Autodesk Inventor part; units mm, degrees
ref_plane "YZ Plane" through (0, 0, 0) normal (1, 0, 0) x (0, 1, 0)
ref_plane "XZ Plane" through (0, 0, 0) normal (0, 1, 0) x (-1, 0, 0)
ref_plane "XY Plane" through (0, 0, 0) normal (0, 0, 1) x (1, 0, 0)
sketch "Sketch1" plane through (0, 0, 0) normal (0, 0, 1) x (1, 0, 0)
  line L0 (-250, 0) -> (250, 0) construction
  line L1 (-250, -50) -> (250, -50)
  line L2 (250, 50) -> (-250, 50)
  arc A0 (-250, 50) -> (-250, -50) centre (-250, 0) ccw
  arc A1 (250, -50) -> (250, 50) centre (250, 0) ccw
  circle A2 centre (-250, 0) radius 25
  circle A3 centre (0, 0) radius 25
  circle A4 centre (250, 0) radius 25
  circle A5 centre (-125, 0) radius 25
  circle A6 centre (125, 0) radius 25
  dimension "d0" = 500
  dimension "d1" = 50
  dimension "d2" = 50
  dimension "d3" = 125
  dimension "d4" = 125
extrude "Extrusion1" add sketch "Sketch1" along normal mid plane 20
properties part number "CE-10.2.1" material "Aluminum 6061"
Part model, mm, in its own coordinate system. Coordinates: 2 decimals unless noted, no trailing zeros. Write each loop counter-clockwise with the first axis right and the second up, starting at its lowest first coordinate (ties: lowest second). Pieces come first, ordered by that corner, then holes.
Item 1: Slice it at C-C (z = 4.5). Write the cut outline in (x, y), and give its area (3 significant figures).
Item 2: Slice it at B-B (y = 0). Write the cut outline in (x, z).
Item 3: Slice it at A-A (x = 125). Write the cut outline in (y, z).
Item 4: Mould opens along Y. For faces 1 (the face through (-4, 34, 10)), 2 (the face through (105, 15, 0)), 3 (the face through (299.988, 1.099, -0.14)), 4 (the face through (273.846, -7.509, -0.14)) say: released by +Y, released by -Y, zero draft, split by the parting line, or undercut.
Item 5: Pin check, flat tips, straight feed: pin 1 (12 mm diameter, centred on y = 10.5, z = -6.5, fed in from +X); pin 2 (12 mm diameter, centred on x = 232.5, y = 3, fed in from +Z); pin 3 (5 mm diameter, centred on y = 5.5, z = 3.5, fed in from +X); pin 4 (1.5 mm diameter, centred on y = -17.5, z = -1.5, fed in from -X). Stop position of each tip, or through.
Item 6: Probe line 1 (Y direction, x = -125, z = -5.75); line 2 (X direction, y = 20, z = 1); line 3 (X direction, y = -11, z = -6) (3 decimals). List the from-to ranges inside material, lowest first.
Item 7: Slice it at D-D (y = 34.5). Write the cut outline in (x, z).
Results found:
1. outline: (-250, -50) - (250, -50) arc R50 ccw to (250, 50) - (-250, 50) arc R50 ccw to start; hole circle Ø50 at (-250, 0); hole circle Ø50 at (-125, 0); hole circle Ø50 at (0, 0); hole circle Ø50 at (125, 0); hole circle Ø50 at (250, 0)
1. area: 48,000 mm2
2. outline: (-300, -10) - (-275, -10) - (-275, 10) - (-300, 10) - close; (-225, -10) - (-150, -10) - (-150, 10) - (-225, 10) - close; (-100, -10) - (-25, -10) - (-25, 10) - (-100, 10) - close; (25, -10) - (100, -10) - (100, 10) - (25, 10) - close; (150, -10) - (225, -10) - (225, 10) - (150, 10) - close; (275, -10) - (300, -10) - (300, 10) - (275, 10) - close
3. outline: (-50, -10) - (-25, -10) - (-25, 10) - (-50, 10) - close; (25, -10) - (50, -10) - (50, 10) - (25, 10) - close
4. face 1: zero draft
4. face 2: undercut
4. face 3: split by the parting line
4. face 4: undercut
5. pin 1: stops at x = 299.8
5. pin 2: passes through
5. pin 3: stops at x = 299.91
5. pin 4: stops at x = -297.11
6. line 1: y = -50 to -25, 25 to 50
6. line 2: x = -295.83 to -265, -235 to -140, -110 to -15, 15 to 110, 140 to 235, 265 to 295.83
6. line 3: x = -298.775 to -272.45, -227.55 to -147.45, -102.55 to -22.45, 22.45 to 102.55, 147.45 to 227.55, 272.45 to 298.775
7. outline: (-286.19, -10) - (286.19, -10) - (286.19, 10) - (-286.19, 10) - close
